Can you work these out from the model? Positions are in its coordinate system, mm. Round coordinates to 2 decimals unless told otherwise and drop trailing zeros. Order: outer loops, then holes, each group sorted by start corner. A loop starts at its lowest first (then second) coordinate and runs counter-clockwise, first axis right, second up. Notation, with made-up numbers: M 15,7.25 L 35,7.25 A24 cw 35,18.25 Z; hole C -4.75,65 d7. An arc over 180 degrees is marked long. One line per question, with ' | ' between items.
Autodesk Inventor part; units mm, degrees
ref_plane "YZ Plane" through (0, 0, 0) normal (1, 0, 0) x (0, 1, 0)
ref_plane "XZ Plane" through (0, 0, 0) normal (0, 1, 0) x (-1, 0, 0)
ref_plane "XY Plane" through (0, 0, 0) normal (0, 0, 1) x (1, 0, 0)
sketch "Sketch1" plane through (0, 0, 0) normal (0, 0, 1) x (1, 0, 0)
  circle A0 centre (9, 9) radius 2.5
  line L0 (200, 18) -> (200, 0)
  line L1 (200, 0) -> (0, 0)
  line L2 (0, 0) -> (0, 200)
  line L3 (0, 200) -> (18, 200)
  line L4 (18, 200) -> (200, 18)
  circle A1 centre (29, 9) radius 2.5
  circle A2 centre (169, 9) radius 2.5
  circle A3 centre (189, 9) radius 2.5
  circle A4 centre (9, 29) radius 2.5
  circle A5 centre (9, 169) radius 2.5
  circle A6 centre (9, 189) radius 2.5
extrude "Extrusion1" add sketch "Sketch1" along normal blind 5
hole "Hole1" at (60, 60, 5) direction (0, 0, -1) diameter 7.75 end through all
properties part number "GUSSET_200MM"
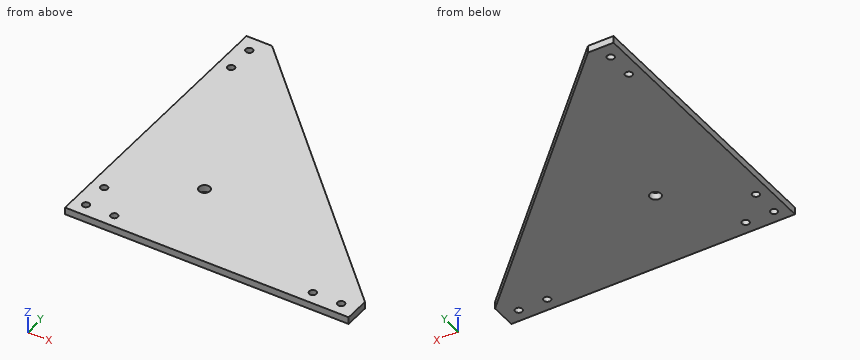
(1) Will these pins go through, and if not, where does the flat tip stop? pin 1 Ø4 at (x, y) = (189, 9) entering from -Z; pin 2 Ø1 at (x, z) = (71, 1) entering from +Y; pin 3 Ø3 at (x, z) = (79, 4.5) entering from +Y.
Final values:
pin 1: through | pin 2: y = 147.5 | pin 3: y = 140.5
(2) If we section it at D-D on y = 9: Please give me the cut outline in (x, z).
Final values:
outline: M 0,0 L 6.5,0 L 6.5,5 L 0,5 Z; M 11.5,0 L 26.5,0 L 26.5,5 L 11.5,5 Z; M 31.5,0 L 166.5,0 L 166.5,5 L 31.5,5 Z; M 171.5,0 L 186.5,0 L 186.5,5 L 171.5,5 Z; M 191.5,0 L 200,0 L 200,5 L 191.5,5 Z
(3) If we section it at C-C on z = 3.35: State how many separate pieces and enclosed holes the cut face has, plus the area to 3 significant figures.
Final values:
separate pieces: 1 | enclosed holes: 8 | area: 23,300 mm^2
(4) Please list where these lines run through material, in increasing order: probe 1 along X at (y, z) = (189, 1.35); probe 2 along X at (y, z) = (190.5, 3.1); probe 3 along Y at (x, z) = (169, 1.9). Write a range as [from, to].
Final values:
probe 1: [0, 6.5], [11.5, 29] | probe 2: [0, 7], [11, 27.5] | probe 3: [0, 6.5], [11.5, 49]
(5) If we section it at A-A on y = 189: Please give me the cut outline in (x, z).
Final values:
outline: M 0,0 L 6.5,0 L 6.5,5 L 0,5 Z; M 11.5,0 L 29,0 L 29,5 L 11.5,5 Z
(6) If we section it at B-B on x = 169: Please give me the cut outline in (y, z), plus the area to 3 significant figures.
Final values:
outline: M 0,0 L 6.5,0 L 6.5,5 L 0,5 Z; M 11.5,0 L 49,0 L 49,5 L 11.5,5 Z | area: 220 mm^2
